Build history of the part. All positions in model axes, mm. A direction names the side the tool comes from. Round coordinates to 2 decimals unless told otherwise and drop trailing zeros. Write each loop counter-clockwise with the first axis right and the second up, starting at its lowest first coordinate (ties: lowest second). Pieces come first, ordered by that corner, then holes. Notation, with made-up numbers: (44, 87.5) -> (101, 87.5) arc R32 ccw to (101, 113.5) -> close; hole circle Ø5 at (41.5, 58.25). An arc over 180 degrees is marked (long way). One line per question, with ' | ' between items.
from build123d import *

# Parameters (mm, degrees)
BOSS_EXTRUDE1_DEPTH = 22
FILLET1_R           = 1
FILLET2_R           = 2
CUT_EXTRUDE1_DEPTH  = 4.256447705


with BuildPart() as part:
    # Sketch1 → Boss-Extrude1 (new body)
    with BuildSketch(Plane.XY):
        Polygon((-37.577345781, 8.579229267), (17.308314067, 8.579229267), (22.382654219, 6.732320493), (21.869624004, 5.322781562), (17.222654219, 7.014140243), (-37.577345781, 7.014140243), align=None)
    extrude(amount=BOSS_EXTRUDE1_DEPTH)

    # Fillet1
    fillet1_edges = [part.edges().sort_by_distance(p)[0] for p in [
        (17.308314067, 8.579229267, 11),
    ]]
    fillet(fillet1_edges, radius=FILLET1_R)

    # Fillet2
    fillet2_edges = [part.edges().sort_by_distance(p)[0] for p in [
        (22.126139112, 6.027551028, 22),
        (-37.577345781, 7.796684755, 22),
        (22.126139112, 6.027551028, 0),
        (-37.577345781, 7.796684755, 0),
    ]]
    fillet(fillet2_edges, radius=FILLET2_R)

    # Sketch3 → Cut-Extrude1 (cut, through all)
    with BuildSketch(Plane(origin=(0, 8.579229267, 0), x_dir=(1, 0, 0), z_dir=(0, 1, 0))):
        with BuildLine():
            Line((-24.077345781, -17), (-24.077345781, -7))
            ThreePointArc((-24.077345781, -7), (-25.827345781, -5.25), (-27.577345781, -7))
            Line((-27.577345781, -7), (-27.577345781, -17))
            ThreePointArc((-27.577345781, -17), (-25.827345781, -18.75), (-24.077345781, -17))
        make_face()
        with BuildLine():
            Line((9.422654219, -17), (9.422654219, -7))
            ThreePointArc((9.422654219, -7), (7.672654219, -5.25), (5.922654219, -7))
            Line((5.922654219, -7), (5.922654219, -17))
            ThreePointArc((5.922654219, -17), (7.672654219, -18.75), (9.422654219, -17))
        make_face()
    extrude(amount=-CUT_EXTRUDE1_DEPTH, mode=Mode.SUBTRACT)


solid = part.part
(1) Slice it at C-C (x = -16). Write the cut outline in (y, z), then the cut area to 3 significant figures.
Calculated:
outline: (7.01, 0) -> (8.58, 0) -> (8.58, 22) -> (7.01, 22) -> close | area: 34.4 mm2
(2) Mould opens along X. For faces 4 (the cylindrical face through (21.557, 6.223, 21.43)), 5 (the flat face through (-7, 8, 0)), 6 (the flat face through (-24.077, 8, 12)), 7 (the flat face through (5.923, 8, 12)) say: pulls with the +X half, pulls with the -X half, needs draft (parallel to the pull), parting line crosses it, or undercut.
Calculated:
face 4: pulls with the +X half | face 5: needs draft | face 6: undercut | face 7: undercut
(3) Slice it at A-A (z = 8.25). Write the cut outline in (x, y).
Calculated:
outline: (-37.58, 7.01) -> (-27.58, 7.01) -> (-27.58, 8.58) -> (-37.58, 8.58) -> close; (-24.08, 7.01) -> (5.92, 7.01) -> (5.92, 8.58) -> (-24.08, 8.58) -> close; (9.42, 7.01) -> (17.22, 7.01) -> (21.87, 5.32) -> (22.38, 6.73) -> (17.47, 8.52) arc R1 ccw to (17.13, 8.58) -> (9.42, 8.58) -> close
(4) Slice it at B-B (y = 7.95). Write the cut outline in (x, z), then the cut area to 3 significant figures.
Calculated:
outline: (-37.58, 2) arc R2 ccw to (-35.58, 0) -> (19.04, 0) -> (19.04, 22) -> (-35.58, 22) arc R2 ccw to (-37.58, 20) -> close; hole (-27.58, 7) arc R1.75 ccw to (-24.08, 7) -> (-24.08, 17) arc R1.75 ccw to (-27.58, 17) -> close; hole (5.92, 7) arc R1.75 ccw to (9.42, 7) -> (9.42, 17) arc R1.75 ccw to (5.92, 17) -> close | area: 1,150 mm2
(5) Wall check: line 1 (Y direction, x = -30, z = 1.25). Give the ranges that are in metal, low to high. Write a range as from..to.
Calculated:
line 1: 7.01..8.58
(6) Drop flat-ended pins along their axis: pin 1 (1.7 mm diameter, centred on y = 7.5, z = 12, fed in from +X); pin 2 (5 mm diameter, centred on x = -5.5, z = 13, fed in from -Y). Give the stop position or say it passes through.
Calculated:
pin 1: x = 22.38 | pin 2: y = 7.01
(7) 3-axis set-ups, long thin cutter, end or side, ignore diameter. For faces 1 (the flat face through (-10, 7.014, 11)), 2 (the cylindrical face through (-25.87, 7.81, 18.75)), 3 (the flat face through (-7, 8, 22)): which of +Z, -Z, +X, -X, +Y, -Y reach the whole face in a straight line?
Calculated:
face 1: +Z, -Z, -X, -Y | face 2: +Y, -Y | face 3: +Z, +X, -X, +Y, -Y
